```python
from build123d import *

# Parameters (mm, degrees)
BOSS_EXTRUDE1_DEPTH = 6
CUT_EXTRUDE1_DEPTH  = 6
CUT_EXTRUDE2_DEPTH  = 1


with BuildPart() as part:
    # Sketch2 → Boss-Extrude1 (new body)
    with BuildSketch(Plane.XY):
        with BuildLine():
            Line((0, 2), (-4, 2))
            Line((-4, 2), (-4, 3))
            Line((-4, 3), (0, 3))
            ThreePointArc((0, 3), (3, 0), (0, -3))
            Line((0, -3), (-2, -3))
            Line((-2, -3), (-2, -2))
            Line((-2, -2), (0, -2))
            ThreePointArc((0, -2), (2, 0), (0, 2))
        make_face()
    extrude(amount=BOSS_EXTRUDE1_DEPTH)

    # Sketch3 → Cut-Extrude1 (cut)
    with BuildSketch(Plane.XZ.offset(-2)):
        Polygon((-2, 6), (-2, 4), (-4, 2), (-4, 6), align=None)
    extrude(amount=-CUT_EXTRUDE1_DEPTH, mode=Mode.SUBTRACT)

    # Sketch4 → Cut-Extrude2 (cut)
    with BuildSketch(Plane.XZ.offset(3)):
        Polygon((0, 6), (-2, 2), (-2, 6), align=None)
    extrude(amount=-CUT_EXTRUDE2_DEPTH, mode=Mode.SUBTRACT)


solid = part.part
```
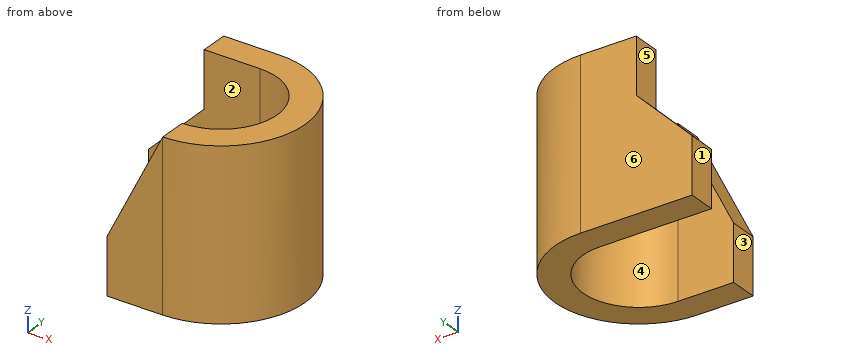
Can you work these out from the model? Positions are in its coordinate system, mm. Face numbers are marked on the shaded views. A direction names the side the tool comes from. Coordinates: 2 decimals unless noted, no trailing zeros. Write each loop counter-clockwise with the first axis right and the second up, starting at its lowest first coordinate (ties: lowest second). Pieces come first, ordered by that corner, then holes. Notation, with made-up numbers: M -37.5,-27.5 L -3.5,-27.5 A7 ccw -3.5,-22.5 Z; hole C -12.5,71 d5. An arc over 180 degrees is marked long. Write item = value, one per line. Start each with the question number.
Q1. If we section it at A-A, the plane x = 0.5: Write out the boundary of the cut face in (y, z), then the cut area to 3 significant figures.
Q2. If we section it at D-D, the plane x = -3.5: Write out the boundary of the cut face in (y, z), then the cut area to 3 significant figures.
Q3. I'm going to push flat-ended pins straight in: pin 1 (2 mm diameter, centred on y = 2, z = 1.5, fed in from +X); pin 2 (0.5 mm diameter, centred on y = -2.5, z = 1.5, fed in from -X). Where does each tip first touch, or does it pass through?
Q4. If we section it at B-B, the plane z = 4.5: Write out the boundary of the cut face in (x, y).
Q5. If we section it at C-C, the plane y = -2.35: Write out the boundary of the cut face in (x, z).
Q6. On a 3-axis mill with a long thin cutter (end or side, diameter ignored), from which of +Z, -Z, +X, -X, +Y, -Y can I reach the whole of each face in a straight line? I mean the marked faces 1, 2 and 3. Say none if no direction works.
Q7. Thinking about a two-plate mould opening in Y: for the marked faces 4, 5 and 6, which applies, released by +Y, released by -Y, zero draft, split by the parting line, or undercut?
Q8. If I drill on L1, parallel to Y at x = -0.5, z = 2.8; L2, parallel to X at y = -0.05, z = 4.35; L3, parallel to Y at x = 1.25, z = 1.25, over which ranges is the centre line in solid material (lowest first)? Write a range as [from, to].
Check sheet entries:
q1.outline = M -2.96,0 L -1.94,0 L -1.94,6 L -2.96,6 Z; M 1.94,0 L 2.96,0 L 2.96,6 L 1.94,6 Z
q1.area = 12.3 mm²
q2.outline = M 2,0 L 3,0 L 3,2.5 L 2,2.5 Z
q2.area = 2.50 mm²
q3.pin_1 = 2.83
q3.pin_2 = -2
q4.outline = M -2,2 L 0,2 A2 cw 0,-2 L -0.75,-2 L -0.75,-3 L 0,-3 A3 ccw 0,3 L -2,3 Z
q5.outline = M -2,0 L 1.86,0 L 1.86,6 L 0,6 L -2,2 Z
q6.face_1 = +Z, -Z, -X, +Y, -Y
q6.face_2 = +Z, -Z, -X
q6.face_3 = +Z, -Z, -X, -Y
q7.face_4 = undercut
q7.face_5 = zero draft
q7.face_6 = released by +Y
q8.L1 = [-3, -2], [2, 3]
q8.L2 = [2, 3]
q8.L3 = [-2.73, -1.56], [1.56, 2.73]
